Part model, mm, in its own coordinate system. A direction names the side the tool comes from. Round coordinates to 2 decimals unless told otherwise and drop trailing zeros. Loops run counter-clockwise (first coordinate to the right, second up) from the corner with the lowest first, then second, coordinate; pieces in that order, holes last.
(1) Probe probe 1 along Z at (x, y) = (-57.5, 0); probe 2 along Z at (x, y) = (-105.25, 0) (3 decimals); probe 3 along X at (y, z) = (1, 22). List the from-to ranges inside material, lowest first.
(2) Flat gauge pins, fed straight in: pin 1 (1.5 mm diameter, centred on x = -43, y = 19, fed in from -Z); pin 2 (11.5 mm diameter, centred on y = 0, z = 29.21, fed in from +X); pin 3 (21 mm diameter, centred on x = -10, z = 16.5, fed in from -Y); pin 4 (7.5 mm diameter, centred on x = -48, z = 24, fed in from -Y). Where does each tip first touch, or does it go through?
(3) Tool access for faces 1 (the face through (-101, 19.05, 21)), 2 (the face through (-130.125, 1.907, 27.62)), 3 (the face through (-66.332, 4.1, 27.6)): list every direction of +Z, -Z, +X, -X, +Y, -Y with a clear straight run to the whole face (end or side of a thin tool).
(4) Cut at C-C on z = 29.21. Count the separate pieces of the cut face and the enclosed holes in it, then the cut area to 3 significant figures.
(5) Mould opens along X. For faces 4 (the face through (-101, 0, 38.1)), 5 (the face through (-101.12, -0.96, 24.87)), 6 (the face through (-155.232, 1, 3)), 7 (the face through (-101, -19.05, 21)) say: +X half, -X half, draft (parallel to the pull), parting line (faces both ways), or undercut.
(6) Cut at A-A on z = 10. List the corners of the cut face in (x, y), then the cut area to 3 significant figures.
from build123d import *

# Parameters (mm, degrees)
F0_W     = 25.4
F0_H     = 12.7
F1_DEPTH = 50.8
F0_R     = 6.35
F0_W_2   = 19.05
F0_H_2   = 38.1
F2_DEPTH = 38.1
F3_DEPTH = 5.08
F5_DEPTH = 25.4
F6_R     = 4.1275
F7_DEPTH = 25.4
F8_R     = 4.445
F9_DEPTH = 25.4


with BuildPart() as f1:
    # F0 (on Top) → F1 (new body)
    with BuildSketch(Plane.XY):
        with Locations((-53.6319812462, 0)):
            Rectangle(F0_W, F0_H)
    extrude(amount=F1_DEPTH)



with BuildPart() as f1b:
    # F0 (on Top) → F1, piece 2 (new body)
    with BuildSketch(Plane.XY):
        with Locations((28.9180187538, 0)):
            Circle(F0_R)
    extrude(amount=F1_DEPTH)


with BuildPart() as f1c:
    # F0 (on Top) → F1, piece 3 (new body)
    with BuildSketch(Plane.XY):
        with Locations((-136.1819812462, 0)):
            Circle(F0_R)
    extrude(amount=F1_DEPTH)


with BuildPart() as f2:
    # F0 (on Top) → F2 (new body)
    with BuildSketch(Plane.XY):
        with Locations((-101.2569812462, 0)):
            Rectangle(F0_W_2, F0_H_2)
    extrude(amount=F2_DEPTH)


with BuildPart() as f2b:
    # F0 (on Top) → F2, piece 2 (new body)
    with BuildSketch(Plane.XY):
        with Locations((-6.0069812462, 0)):
            Rectangle(F0_W_2, F0_H_2)
    extrude(amount=F2_DEPTH)


with BuildPart() as f1_1:
    add(f1.part)

    add(f1b.part)  # F3 merges F1b

    add(f1c.part)  # F3 merges F1c

    add(f2.part)  # F3 merges F2

    add(f2b.part)  # F3 merges F2b
    # F0 (on Top) → F3 (join)
    with BuildSketch(Plane.XY):
        Polygon((47.9680187538, 38.1), (-155.2319812462, 38.1), (-155.2319812462, -38.1), (47.9680187538, -38.1), (47.9680187538, 0), align=None)
        with Locations((-136.1819812462, 0)):
            Circle(F0_R, mode=Mode.SUBTRACT)
        with Locations((-101.2569812462, 0)):
            Rectangle(F0_W_2, F0_H_2, mode=Mode.SUBTRACT)
        with Locations((-53.6319812462, 0)):
            Rectangle(F0_W, F0_H, mode=Mode.SUBTRACT)
        with Locations((-6.0069812462, 0)):
            Rectangle(F0_W_2, F0_H_2, mode=Mode.SUBTRACT)
        with Locations((28.9180187538, 0)):
            Circle(F0_R, mode=Mode.SUBTRACT)
    extrude(amount=F3_DEPTH)

    # F4 (on face) → F5 (cut)
    with BuildSketch(Plane.YZ.offset(3.5180187538)):
        with BuildLine():
            ThreePointArc((0, 33.9725), (-3.3675960454, 25.8424039546), (4.7625, 29.21))
            ThreePointArc((4.7625, 29.21), (3.3675960454, 32.5775960454), (0, 33.9725))
        make_face()
    extrude(amount=-F5_DEPTH, mode=Mode.SUBTRACT)

    # F6 (on face) → F7 (cut)
    with BuildSketch(Plane.YZ.offset(-40.9319812462)):
        with Locations((0, 29.21)):
            Circle(F6_R)
    extrude(amount=-F7_DEPTH, mode=Mode.SUBTRACT)

    # F8 (on face) → F9 (cut)
    with BuildSketch(Plane.YZ.offset(-91.7319812462)):
        with Locations((0, 29.21)):
            Circle(F8_R)
    extrude(amount=-F9_DEPTH, mode=Mode.SUBTRACT)


solid = f1_1.part
Final values:
1. probe 1: z = 0 to 25.08, 33.34 to 50.8
1. probe 2: z = 0 to 24.765, 33.655 to 38.1
1. probe 3: x = -142.45 to -129.91, -110.78 to -91.73, -66.33 to -40.93, -15.53 to 3.52, 22.65 to 35.19
2. pin 1: stops at z = 0
2. pin 2: stops at x = 35.27
2. pin 3: stops at y = -19.05
2. pin 4: stops at y = -6.35
3. face 1: +Z, +X, -X, +Y
3. face 2: +Z
3. face 3: +Z, +Y, -Y
4. separate pieces: 8
4. enclosed holes: 0
4. area: 1,470 mm2
5. face 4: undercut
5. face 5: undercut
5. face 6: -X half
5. face 7: draft
6. outline: circle Ø12.7 at (-136.18, 0); (-110.78, -19.05) - (-91.73, -19.05) - (-91.73, 19.05) - (-110.78, 19.05) - close; (-66.33, -6.35) - (-40.93, -6.35) - (-40.93, 6.35) - (-66.33, 6.35) - close; (-15.53, -19.05) - (3.52, -19.05) - (3.52, 19.05) - (-15.53, 19.05) - close; circle Ø12.7 at (28.92, 0)
6. area: 2,030 mm2
